Part print with two shaded views. Sizes in mm from the minimum x, y, z corner. Round coordinates to 2 decimals unless told otherwise and drop trailing zeros. Order: outer loops, then holes, each group sorted by start corner. A loop starts at its lowest first (then second) coordinate and runs counter-clockwise, first axis right, second up. Notation, with made-up numbers: M 28.25,-31.5 L 52.25,-31.5 A28 cw 52.25,1.5 Z; hole C 1,-12 d3. An arc over 180 degrees is marked long. One line per question, with ' | ' between items.
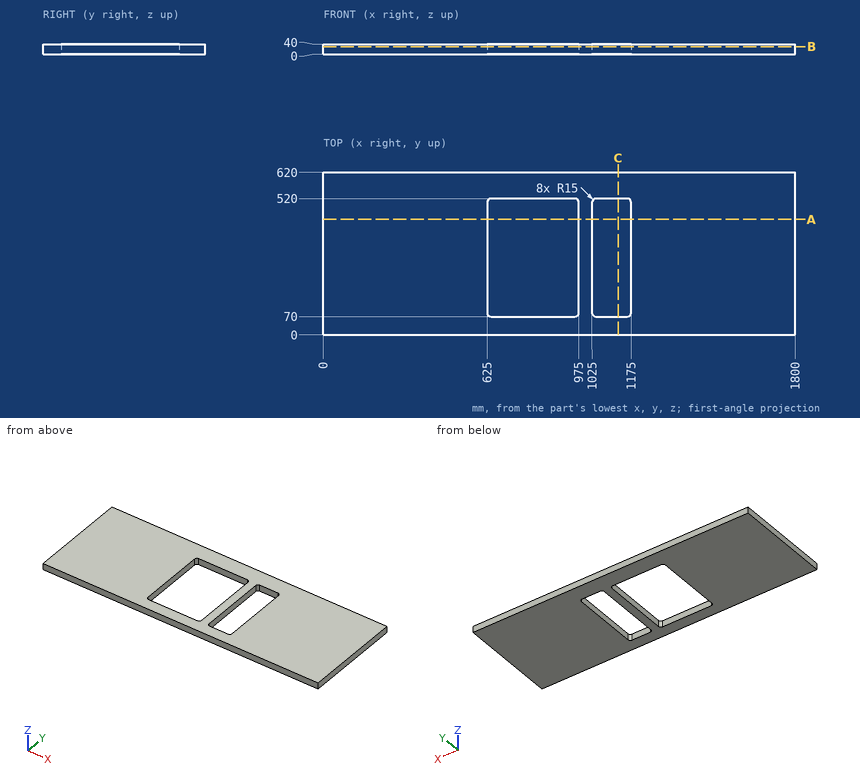
1) Saw through at B-B (z = 30). List the corners of the cut face in (x, y), plus the area to 3 significant figures.
The answers:
outline: M 0,0 L 1800,0 L 1800,620 L 0,620 Z; hole M 625,85 A15 ccw 640,70 L 960,70 A15 ccw 975,85 L 975,505 A15 ccw 960,520 L 640,520 A15 ccw 625,505 Z; hole M 1025,85 A15 ccw 1040,70 L 1160,70 A15 ccw 1175,85 L 1175,505 A15 ccw 1160,520 L 1040,520 A15 ccw 1025,505 Z | area: 891,000 mm²
2) Probe line 1 (X direction, y = 97, z = 33); line 2 (Y direction, x = 1146, z = 7); line 3 (X direction, y = 79, z = 11). List the from-to ranges inside material, lowest first. Write a range as [from, to].
The answers:
line 1: x = [0, 625], [975, 1025], [1175, 1800] | line 2: y = [0, 70], [520, 620] | line 3: x = [0, 626.25], [973.75, 1026.25], [1173.75, 1800]
3) Saw through at C-C (x = 1125). List the corners of the cut face in (y, z).
The answers:
outline: M 0,0 L 70,0 L 70,40 L 0,40 Z; M 520,0 L 620,0 L 620,40 L 520,40 Z
4) Saw through at A-A (y = 441). List the corners of the cut face in (x, z), plus the area to 3 significant figures.
The answers:
outline: M 0,0 L 625,0 L 625,40 L 0,40 Z; M 975,0 L 1025,0 L 1025,40 L 975,40 Z; M 1175,0 L 1800,0 L 1800,40 L 1175,40 Z | area: 52,000 mm²
